Job drawing, mm, ordinate dimensions from the low corner. One solid piece. Round coordinates to 2 decimals unless told otherwise and drop trailing zeros. Write each loop counter-clockwise with the first axis right and the second up, starting at its lowest first coordinate (ties: lowest second). Pieces come first, ordered by that corner, then holes.
1) Flat gauge pins, fed straight in: pin 1 (10 mm diameter, centred on y = 35, z = 17, fed in from -X); pin 2 (1.5 mm diameter, centred on y = 30.5, z = 5.5, fed in from +X); pin 3 (2.5 mm diameter, centred on y = 50.5, z = 11.5, fed in from +X). Where does each tip first touch, or does it go through?
2) Saw through at D-D on z = 4. Write the cut outline in (x, y).
3) Saw through at B-B on z = 12.5. Count the separate pieces of the cut face and the enclosed holes in it, and give its area (3 significant figures).
4) Drill centre lines: L1, parallel to Y at x = 7, z = 5.25; L2, parallel to Y at x = 44.45, z = 12.5; L3, parallel to Y at x = 0.8, z = 12.5. Where is each one in solid material? Low to high.
5) Saw through at A-A on y = 33.5. Write the cut outline in (x, z).
6) Saw through at C-C on x = 29. Write the cut outline in (y, z), and give its area (3 significant figures).
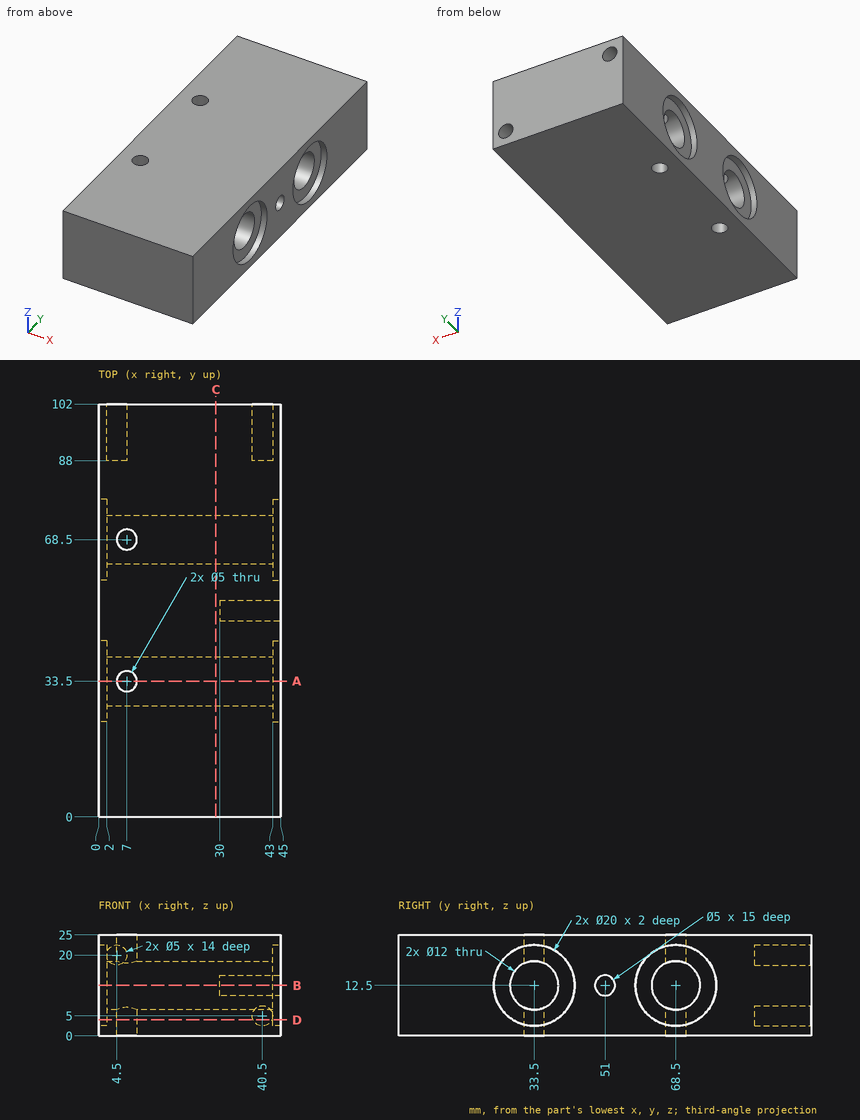
Completed:
1. pin 1: stops at x = 2
1. pin 2: stops at x = 43
1. pin 3: stops at x = 30
2. outline: (0, 0) - (45, 0) - (45, 28.23) - (43, 28.23) - (43, 38.77) - (45, 38.77) - (45, 63.23) - (43, 63.23) - (43, 73.77) - (45, 73.77) - (45, 102) - (42.79, 102) - (42.79, 88) - (38.21, 88) - (38.21, 102) - (0, 102) - (0, 73.77) - (2, 73.77) - (2, 63.23) - (0, 63.23) - (0, 38.77) - (2, 38.77) - (2, 28.23) - (0, 28.23) - close; hole circle Ø5 at (7, 33.5); hole circle Ø5 at (7, 68.5)
3. separate pieces: 3
3. enclosed holes: 0
3. area: 3,370 mm2
4. L1: y = 0 to 31, 36 to 66, 71 to 102
4. L2: y = 0 to 23.5, 43.5 to 48.5, 53.5 to 58.5, 78.5 to 102
4. L3: y = 0 to 23.5, 43.5 to 58.5, 78.5 to 102
5. outline: (0, 0) - (4.5, 0) - (4.5, 6.5) - (2, 6.5) - (2, 2.5) - (0, 2.5) - close; (0, 22.5) - (2, 22.5) - (2, 18.5) - (4.5, 18.5) - (4.5, 25) - (0, 25) - close; (9.5, 0) - (45, 0) - (45, 2.5) - (43, 2.5) - (43, 6.5) - (9.5, 6.5) - close; (9.5, 18.5) - (43, 18.5) - (43, 22.5) - (45, 22.5) - (45, 25) - (9.5, 25) - close
6. outline: (0, 0) - (102, 0) - (102, 25) - (0, 25) - close; hole circle Ø12 at (33.5, 12.5); hole circle Ø12 at (68.5, 12.5)
6. area: 2,320 mm2
